from build123d import *

# Parameters (mm, degrees)
F0_W     = 33
F0_H     = 13
F0_W_2   = 3.5
F0_H_2   = 5
F0_W_3   = 15
F1_DEPTH = 13.04
F2_W     = 33
F2_H     = 4
F3_DEPTH = 40.6
F4_R     = 2.5
F5_R     = 2.5
F6_DEPTH = 9.9
F4_R_2   = 5
F5_R_2   = 5
F7_DEPTH = 3
F8_R     = 5


with BuildPart() as f1:
    # F0 (on Top) → F1 (new body)
    with BuildSketch(Plane.XY):
        with Locations((0, 2.5)):
            Rectangle(F0_W, F0_H)
        with Locations((-18.25, 2.5)):
            Rectangle(F0_W_2, F0_H)
        Polygon((16.5, -4), (-16.5, -4), (-16.5, -9), (0, -9), (16.5, -9), align=None)
        with Locations((-18.25, -6.5)):
            Rectangle(F0_W_2, F0_H_2)
        with Locations((-27.5, -6.5)):
            Rectangle(F0_W_3, F0_H_2)
        with Locations((18.25, 2.5)):
            Rectangle(F0_W_2, F0_H)
        with Locations((18.25, -6.5)):
            Rectangle(F0_W_2, F0_H_2)
        with Locations((27.5, -6.5)):
            Rectangle(F0_W_3, F0_H_2)
    extrude(amount=F1_DEPTH)

    # F2 (on face) → F3 (cut)
    with BuildSketch(Plane(origin=(0, 9, 0), x_dir=(-1, 0, 0), z_dir=(0, 1, 0))):
        with Locations((0, 6.52)):
            Rectangle(F2_W, F2_H)
    extrude(amount=-F3_DEPTH, mode=Mode.SUBTRACT)

    # F4 (on face) + F5 (on face) → F6 (cut)
    with BuildSketch(Plane(origin=(0, -4, 0), x_dir=(-1, 0, 0), z_dir=(0, 1, 0))):
        with Locations((-28, 6.52)):
            Circle(F4_R)
    with BuildSketch(Plane(origin=(0, -4, 0), x_dir=(-1, 0, 0), z_dir=(0, 1, 0))):
        with Locations((28, 6.52)):
            Circle(F5_R)
    extrude(amount=-F6_DEPTH, mode=Mode.SUBTRACT)

    # F4 (on face) + F5 (on face) → F7 (cut)
    with BuildSketch(Plane(origin=(0, -4, 0), x_dir=(-1, 0, 0), z_dir=(0, 1, 0))):
        with Locations((-28, 6.52)):
            Circle(F4_R_2)
        with Locations((-28, 6.52)):
            Circle(F4_R, mode=Mode.SUBTRACT)
    with BuildSketch(Plane(origin=(0, -4, 0), x_dir=(-1, 0, 0), z_dir=(0, 1, 0))):
        with Locations((28, 6.52)):
            Circle(F5_R_2)
        with Locations((28, 6.52)):
            Circle(F5_R, mode=Mode.SUBTRACT)
    extrude(amount=-F7_DEPTH, mode=Mode.SUBTRACT)

    # F8
    f8_edges = [f1.edges().sort_by_distance(p)[0] for p in [
        (35, -6.5, 13.04),
        (35, -6.5, 0),
        (-35, -6.5, 13.04),
        (-35, -6.5, 0),
        (20, 2.5, 13.04),
        (-20, 2.5, 13.04),
        (-20, 2.5, 0),
        (20, 2.5, 0),
    ]]
    fillet(f8_edges, radius=F8_R)


solid = f1.part
Read the model definition and answer for the solid it produces. Units are mm, in the model's axes. A direction names the side the tool comes from. Round coordinates to 2 decimals unless told otherwise and drop trailing zeros. Loops run counter-clockwise (first coordinate to the right, second up) from the corner with the lowest first, then second, coordinate; pieces in that order, holes last.
Q1. Each of these flat-tipped pins is pushed along its axis until it touches: pin 1 (1.5 mm diameter, centred on x = -22, y = -3.5, fed in from +Z); pin 2 (6 mm diameter, centred on x = -28, z = 6.52, fed in from +Y); pin 3 (3 mm diameter, centred on y = -0.5, z = 6, fed in from -X); pin 4 (1.5 mm diameter, centred on y = 4.5, z = 6.5, fed in from +X). Where does it stop, or does it pass through?
Q2. Section D-D on y = -1 is taken. Write down the section's boundary in (x, z).
Q3. Determine the mould class of faces 4 (the face through (0, -9, 9)), 5 (the face through (-16.5, 0, 6)), 6 (the face through (0, -2, 13.04)) for opening direction Z: released by +Z, released by -Z, zero draft, split by the parting line, or undercut.
Q4. Consider probe 1 along X at (y, z) = (-7.75, 6.25); probe 2 along Z at (x, y) = (-2, -3.5); probe 3 along X at (y, z) = (5, 6.5). Determine where each line is inside the solid, lowest interval first.
Q5. Which of the six approach directions +Z, -Z, +X, -X, +Y, -Y give full straight-line access (tool end or side, diameter ignored) to faces 1 (the face through (16.5, 0, 6)), 2 (the face through (32.995, -5.479, 6.74)), 3 (the face through (-18.57, 2.41, 11.54))?
Q6. Section A-A on x = -6 is taken. Write down the section's boundary in (y, z).
Q7. Section C-C on y = -5.5 is taken. Write down the section's boundary in (x, z).
Q8. Section B-B on z = 6.52 is taken. Write down the section's boundary in (x, y).
Output:
1. pin 1: stops at z = 13.04
1. pin 2: stops at y = -7
1. pin 3: stops at x = -20
1. pin 4: stops at x = 20
2. outline: (-20, 5) arc R5 ccw to (-15, 0) - (15, 0) arc R5 ccw to (20, 5) - (20, 8.04) arc R5 ccw to (15, 13.04) - (-15, 13.04) arc R5 ccw to (-20, 8.04) - close; hole (-16.5, 4.52) - (16.5, 4.52) - (16.5, 8.52) - (-16.5, 8.52) - close
3. face 4: zero draft
3. face 5: undercut
3. face 6: released by +Z
4. probe 1: x = -35 to -30.49, -25.51 to -16.5, 16.5 to 25.51, 30.49 to 35
4. probe 2: z = 0 to 4.52, 8.52 to 13.04
4. probe 3: x = -20 to -16.5, 16.5 to 20
5. face 1: +Y, -Y
5. face 2: +Y
5. face 3: +Z, -X, +Y
6. outline: (-9, 0) - (9, 0) - (9, 4.52) - (-9, 4.52) - close; (-9, 8.52) - (9, 8.52) - (9, 13.04) - (-9, 13.04) - close
7. outline: (-35, 5) arc R5 ccw to (-30, 0) - (30, 0) arc R5 ccw to (35, 5) - (35, 8.04) arc R5 ccw to (30, 13.04) - (-30, 13.04) arc R5 ccw to (-35, 8.04) - close; hole circle Ø10 at (-28, 6.52); hole (-16.5, 4.52) - (16.5, 4.52) - (16.5, 8.52) - (-16.5, 8.52) - close; hole circle Ø10 at (28, 6.52)
8. outline: (-35, -9) - (-30.5, -9) - (-30.5, -7) - (-33, -7) - (-33, -4) - (-35, -4) - close; (-25.5, -9) - (-16.5, -9) - (-16.5, 9) - (-20, 9) - (-20, -4) - (-23, -4) - (-23, -7) - (-25.5, -7) - close; (16.5, -9) - (25.5, -9) - (25.5, -7) - (23, -7) - (23, -4) - (20, -4) - (20, 9) - (16.5, 9) - close; (30.5, -9) - (35, -9) - (35, -4) - (33, -4) - (33, -7) - (30.5, -7) - close
